Check sheet for the modelled part. Datum: model origin and axes. Units: mm. Round coordinates to 2 decimals unless told otherwise and drop trailing zeros. Loops run counter-clockwise (first coordinate to the right, second up) from the corner with the lowest first, then second, coordinate; pieces in that order, holes last. Notation, with made-up numbers: (-27, 7.25) - (0, 7.25) arc R9 cw to (0, 21.25) - close; hole circle Ø4 at (48, 41). An arc over 180 degrees is marked (long way). Answer in a Markdown table with one row per item. Add a question column.
(1) Cross-section at C-C on z = 12.5. Enter the section's corners in (x, y).
(2) Mould release check, pull along Y, two halves, no side actions. Record for faces 1 (the cylindrical face through (-0.867, 3.905, 29.584)), 2 (the flat face through (-1, 3, 60)), 3 (the cylindrical face through (-0.54, 2.44, 29.58)): +Y half, -Y half, draft (parallel to the pull), parting line (faces both ways), or undercut.
(3) Thickness scan on line 1 along Y through (x, z) = (0, 41.5); line 2 along Y through (x, z) = (-0.5, 13.5); line 3 along X through (y, z) = (-1.5, 30). Record the ranges inside material, lowest first.
(4) Gauge pin test, flat ends, axial feed: pin 1 (2 mm diameter, centred on y = -2.5, z = 22, fed in from -X); pin 2 (1 mm diameter, centred on y = 2.5, z = 51, fed in from +X). Record the tip position at first contact, or that the pin passes through.
(5) Cross-section at A-A on y = 0. Enter the section's corners in (x, z).
Autodesk Inventor part; units mm, degrees
ref_plane "YZ Plane" through (0, 0, 0) normal (1, 0, 0) x (0, 1, 0)
ref_plane "XZ Plane" through (0, 0, 0) normal (0, 1, 0) x (-1, 0, 0)
ref_plane "XY Plane" through (0, 0, 0) normal (0, 0, 1) x (1, 0, 0)
sketch "Sketch1" plane through (0, 0, 0) normal (0, 0, 1) x (1, 0, 0)
  circle A0 centre (0, 0) radius 4
  circle A1 centre (0, 0) radius 2.5
  dimension "d0" = 8
  dimension "d1" = 5
extrude "Extrusion1" add sketch "Sketch1" along normal blind 60
chamfer "Chamfer1" distance 0.25 angle 45 4 edges at (-4, 0, 0) (-4, 0, 60) (-2.5, 0, 0) (-2.5, 0, 60)
thread "Thread1"
thread "Thread2"
properties part number "60mm M5 Standoff" material "Aluminum 6061"
Answers:
| question | item | result |
|---|---|---|
| 1 | outline | circle Ø8 at (0, 0); hole circle Ø5 at (0, 0) |
| 2 | face 1 | parting line |
| 2 | face 2 | draft |
| 2 | face 3 | undercut |
| 3 | line 1 | y = -4 to -2.5, 2.5 to 4 |
| 3 | line 2 | y = -3.97 to -2.45, 2.45 to 3.97 |
| 3 | line 3 | x = -3.71 to -2, 2 to 3.71 |
| 4 | pin 1 | stops at x = -3.71 |
| 4 | pin 2 | stops at x = 3.46 |
| 5 | outline | (-4, 0.25) - (-3.75, 0) - (-2.75, 0) - (-2.5, 0.25) - (-2.5, 59.75) - (-2.75, 60) - (-3.75, 60) - (-4, 59.75) - close; (2.5, 0.25) - (2.75, 0) - (3.75, 0) - (4, 0.25) - (4, 59.75) - (3.75, 60) - (2.75, 60) - (2.5, 59.75) - close |
